```python
from build123d import *

# Parameters (mm, degrees)
F0_R     = 50.8
F0_R_2   = 6.565866
F0_R_3   = 25.4
F1_DEPTH = 7.9375


with BuildPart() as f1:
    # F0 (on Front) → F1 (new body, symmetric)
    with BuildSketch(Plane.XZ):
        Circle(F0_R)
        with Locations((0, -38.1)):
            Circle(F0_R_2, mode=Mode.SUBTRACT)
        with Locations((-32.995568, -19.05)):
            Circle(F0_R_2, mode=Mode.SUBTRACT)
        Circle(F0_R_3, mode=Mode.SUBTRACT)
        with Locations((32.995568, -19.05)):
            Circle(F0_R_2, mode=Mode.SUBTRACT)
        with Locations((-32.995568, 19.05)):
            Circle(F0_R_2, mode=Mode.SUBTRACT)
        with Locations((0, 38.1)):
            Circle(F0_R_2, mode=Mode.SUBTRACT)
        with Locations((32.995568, 19.05)):
            Circle(F0_R_2, mode=Mode.SUBTRACT)
    extrude(amount=F1_DEPTH, both=True)


solid = f1.part
```
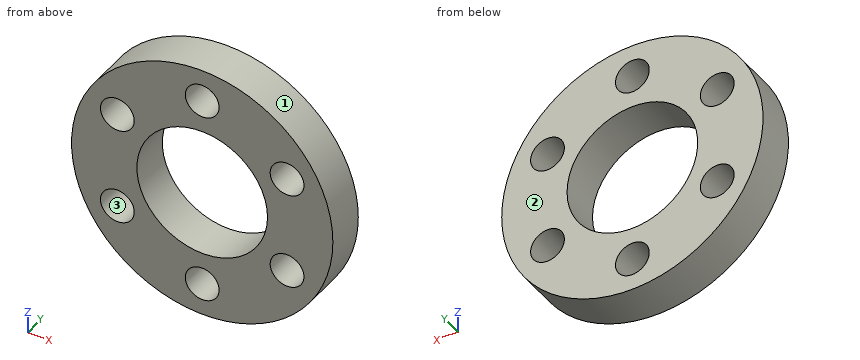
Geometry check sheet. Reference: the model listing, model coordinates, mm. Face numbers are marked on the shaded views. Round coordinates to 2 decimals unless told otherwise and drop trailing zeros. Order: outer loops, then holes, each group sorted by start corner. A loop starts at its lowest first (then second) coordinate and runs counter-clockwise, first axis right, second up. Notation, with made-up numbers: M -3,30.25 L 44,30.25 A12 ccw 44,48.25 Z; hole C 20.5,19 d1. An arc over 180 degrees is marked long. Write item = value, one per line.
Q1. Section check D-D (x = 36). Enter the section's corners in (y, z).
Answer block:
outline = M -7.94,-35.84 L 7.94,-35.84 L 7.94,-24.89 L -7.94,-24.89 Z; M -7.94,-13.21 L 7.94,-13.21 L 7.94,13.21 L -7.94,13.21 Z; M -7.94,24.89 L 7.94,24.89 L 7.94,35.84 L -7.94,35.84 Z
Q2. Section check A-A (y = -1). Enter the section's corners in (x, z), plus the area to 3 significant figures.
Answer block:
outline = C 0,0 d101.6; hole C -33,-19.05 d13.13; hole C -33,19.05 d13.13; hole C 0,0 d50.8; hole C 0,-38.1 d13.13; hole C 0,38.1 d13.13; hole C 33,-19.05 d13.13; hole C 33,19.05 d13.13
area = 5,270 mm^2
Q3. Section check C-C (z = 38.1). Enter the section's corners in (x, y), plus the area to 3 significant figures.
Answer block:
outline = M -33.6,-7.94 L -6.57,-7.94 L -6.57,7.94 L -33.6,7.94 Z; M 6.57,-7.94 L 33.6,-7.94 L 33.6,7.94 L 6.57,7.94 Z
area = 858 mm^2
Q4. Release check for a two-part mould opening along Z. For the marked faces 1, 2 and 3 record: released by +Z, released by -Z, zero draft, split by the parting line, or undercut.
Answer block:
face_1 = split by the parting line
face_2 = zero draft
face_3 = undercut
Q5. Section check B-B (x = 0). Enter the section's corners in (y, z).
Answer block:
outline = M -7.94,-50.8 L 7.94,-50.8 L 7.94,-44.67 L -7.94,-44.67 Z; M -7.94,-31.53 L 7.94,-31.53 L 7.94,-25.4 L -7.94,-25.4 Z; M -7.94,25.4 L 7.94,25.4 L 7.94,31.53 L -7.94,31.53 Z; M -7.94,44.67 L 7.94,44.67 L 7.94,50.8 L -7.94,50.8 Z
Q6. Scan lines: line 1 (Z direction, x = 0, y = 3.5); line 2 (Z direction, x = -5.5, y = 6.5); line 3 (X direction, y = -1.25, z = 16.5). Record each from-to range of solid material in increasing order.
Answer block:
line_1 = -50.8 to -44.67, -31.53 to -25.4, 25.4 to 31.53, 44.67 to 50.8
line_2 = -50.5 to -41.69, -34.51 to -24.8, 24.8 to 34.51, 41.69 to 50.5
line_3 = -48.05 to -39.05, -26.95 to -19.31, 19.31 to 26.95, 39.05 to 48.05
Q7. Depth check by flat-ended pin: pin 1 Ø1 at (y, z) = (-0.5, -20) entering from +X; pin 2 Ø6 at (x, y) = (-9.5, -5.5) entering from -Z; pin 3 Ø1.5 at (y, z) = (2.5, -4.5) entering from +X; pin 4 Ø6 at (x, z) = (-37, 24) entering from +Y. Enter the tip coordinate at first touch or a pass-through.
Answer block:
pin_1 = 46.91
pin_2 = -50.38
pin_3 = 50.66
pin_4 = 7.94
